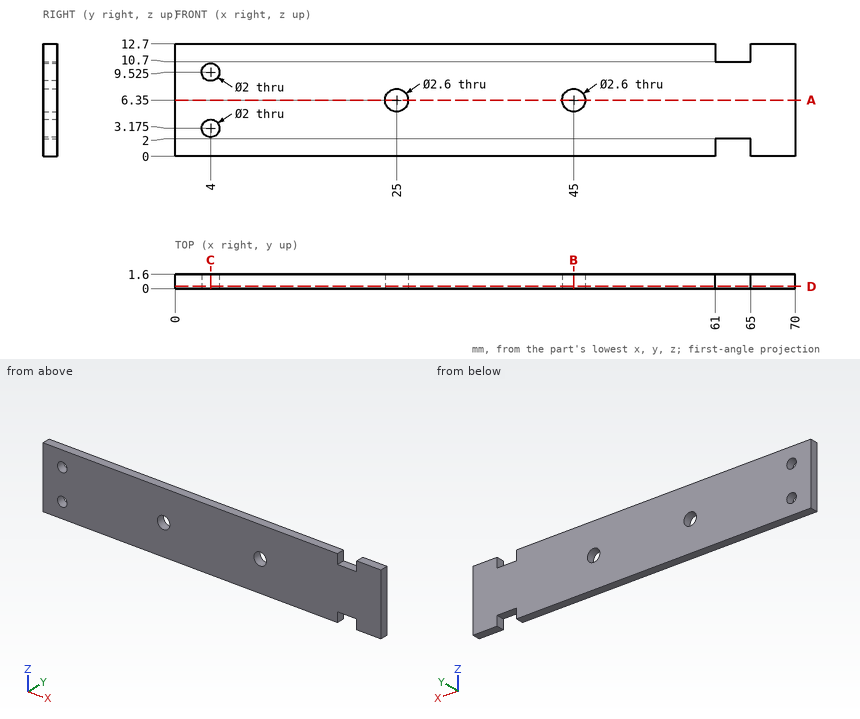
Study the drawing (mm; zero at the part's minimum x, y, z) and answer. Coordinates: 2 decimals unless noted, no trailing zeros. Write each loop counter-clockwise with the first axis right and the second up, starting at its lowest first coordinate (ties: lowest second). Pieces come first, ordered by that corner, then holes.
Q1. A cutting plane is placed at A-A, the plane z = 6.35. Give the vertices of the cut face in (x, y), then the cut area to 3 significant figures.
Q2. A cutting plane is placed at B-B, the plane x = 45. Give the vertices of the cut face in (y, z), then the cut area to 3 significant figures.
Q3. Each of these flat-tipped pins is pushed along its axis until it touches: pin 1 Ø0.8 at (y, z) = (1, 12) entering from -X; pin 2 Ø0.8 at (x, y) = (63.5, 0.5) entering from -Z; pin 3 Ø0.8 at (x, y) = (63.5, 1) entering from +Z. Where does it stop, or does it pass through?
Q4. A cutting plane is placed at D-D, the plane y = 0.25. Give the vertices of the cut face in (x, z) (3 decimals), then the cut area to 3 significant figures.
Q5. A cutting plane is placed at C-C, the plane x = 4. Give the vertices of the cut face in (y, z) (3 decimals), then the cut area to 3 significant figures.
Q6. Find the intervals of material crossed by line 1 (X direction, y = 1.2, z = 6.35); line 2 (Z direction, x = 45, y = 0.95); line 3 (X direction, y = 0.6, z = 1.25), in increasing order.
Findings below:
1. outline: (0, 0) - (23.7, 0) - (23.7, 1.6) - (0, 1.6) - close; (26.3, 0) - (43.7, 0) - (43.7, 1.6) - (26.3, 1.6) - close; (46.3, 0) - (70, 0) - (70, 1.6) - (46.3, 1.6) - close
1. area: 104 mm2
2. outline: (0, 0) - (1.6, 0) - (1.6, 5.05) - (0, 5.05) - close; (0, 7.65) - (1.6, 7.65) - (1.6, 12.7) - (0, 12.7) - close
2. area: 16.2 mm2
3. pin 1: stops at x = 0
3. pin 2: stops at z = 2
3. pin 3: stops at z = 10.7
4. outline: (0, 0) - (61, 0) - (61, 2) - (65, 2) - (65, 0) - (70, 0) - (70, 12.7) - (65, 12.7) - (65, 10.7) - (61, 10.7) - (61, 12.7) - (0, 12.7) - close; hole circle Ø2 at (4, 3.175); hole circle Ø2 at (4, 9.525); hole circle Ø2.6 at (25, 6.35); hole circle Ø2.6 at (45, 6.35)
4. area: 856 mm2
5. outline: (0, 0) - (1.6, 0) - (1.6, 2.175) - (0, 2.175) - close; (0, 4.175) - (1.6, 4.175) - (1.6, 8.525) - (0, 8.525) - close; (0, 10.525) - (1.6, 10.525) - (1.6, 12.7) - (0, 12.7) - close
5. area: 13.9 mm2
6. line 1: x = 0 to 23.7, 26.3 to 43.7, 46.3 to 70
6. line 2: z = 0 to 5.05, 7.65 to 12.7
6. line 3: x = 0 to 61, 65 to 70
